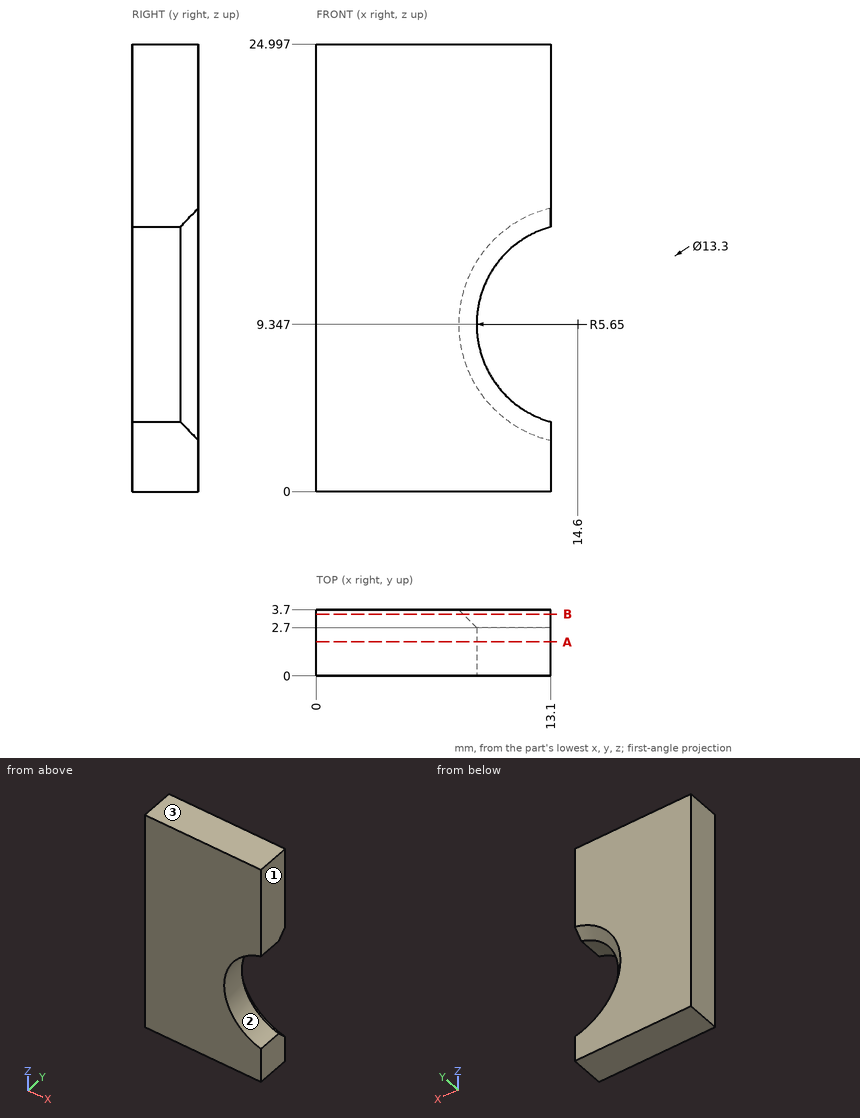
Check sheet for the drawn part. Datum: minimum x, y, z corner. Units: mm. Coordinates: 2 decimals unless noted, no trailing zeros. Order: outer loops, then holes, each group sorted by start corner. A loop starts at its lowest first (then second) coordinate and runs counter-clockwise, first axis right, second up. Notation, with made-up numbers: (-35, 78) -> (-24, 78) arc R15 ccw to (-24, 88) -> close; hole circle Ø7 at (46.25, 37.25). An arc over 180 degrees is marked (long way). Use a Markdown table: item, result. Add a question column.
1. Cross-section at A-A (y = 1.9). Enter the section's corners in (x, z), and give its area (3 significant figures).
2. Cross-section at B-B (y = 3.45). Enter the section's corners in (x, z), and give its area (3 significant figures).
3. Mould release check, pull along Z, two halves, no side actions. Record for the marked faces 1, 2 and 3: pulls with the +Z half, pulls with the -Z half, needs draft (parallel to the pull), parting line crosses it, or undercut.
4. Go/stop test with a flat-tipped pin: pin 1 Ø1.5 at (x, y) = (5, 3) entering from -Z. Record where the tip stops, or that it passes through.
5. Material ranges on L1, parallel to Z at x = 10.5, y = 3 (1 decimal); L2, parallel to Z at x = 12, y = 2.5; L3, parallel to X at y = 0.95, z = 13.5, recorded low to high.
Filled sheet:
| question | item | result |
|---|---|---|
| 1 | outline | (0, 0) -> (13.1, 0) -> (13.1, 3.9) arc R5.65 cw to (13.1, 14.79) -> (13.1, 25) -> (0, 25) -> close |
| 1 | area | 294 mm2 |
| 2 | outline | (0, 0) -> (13.1, 0) -> (13.1, 3.13) arc R6.4 cw to (13.1, 15.57) -> (13.1, 25) -> (0, 25) -> close |
| 2 | area | 282 mm2 |
| 3 | face 1 | needs draft |
| 3 | face 2 | undercut |
| 3 | face 3 | pulls with the +Z half |
| 4 | pin 1 | z = 0 |
| 5 | L1 | 0 to 5, 13.7 to 25 |
| 5 | L2 | 0 to 4.33, 14.36 to 25 |
| 5 | L3 | 0 to 10.77 |
